Read the model definition and answer for the solid it produces. Units are mm, in the model's axes. Face numbers are marked on the shaded views. A direction names the side the tool comes from. Coordinates: 2 decimals unless noted, no trailing zeros. Write each loop counter-clockwise with the first axis right and the second up, starting at its lowest first coordinate (ties: lowest second). Pieces come first, ordered by that corner, then holes. Notation, with made-up numbers: (-13, -19.75) -> (0, -19.75) arc R26 cw to (0, -5.75) -> close; hole circle Ø11 at (21, 27). An arc over 180 degrees is marked (long way). Answer as a JSON object with one key per item and string values. Group by question number.
(1) Flat-ended cylindrical pins translate along their axes: P1, Ø4, axis at x = 36.5, y = 36, coming from the +Z side; P2, Ø2, axis at x = -17, z = 1, coming from the -Y side; P3, Ø1, axis at y = -8.5, z = 1.5, coming from the -X side. Find the tip coordinate at first contact, or state that the pin passes through.
(2) Find section D-D (z = 6.75). Give the vertices of the cut face in (x, y).
(3) Straight lines are drawn through the part: L1, parallel to Y at x = -37.5, z = 2.5; L2, parallel to Y at x = 37.5, z = 6.75; L3, parallel to X at y = 37.5, z = 3.6. For each, find the intervals that lie inside material, in ascending order.
(4) Find section C-C (z = 1.5). Give the vertices of the cut face in (x, y).
(5) Which of the six approach directions +Z, -Z, +X, -X, +Y, -Y give full straight-line access (tool end or side, diameter ignored) to the marked faces 3 and 4?
(6) For a pull along X with two mould halves and no side action, classify the marked faces 1 and 2 as +X half, -X half, draft (parallel to the pull), parting line (faces both ways), or undercut.
(7) Find section A-A (y = 37.5). Give the vertices of the cut face in (x, z).
(8) Find section B-B (x = -37.5). Give the vertices of the cut face in (y, z).
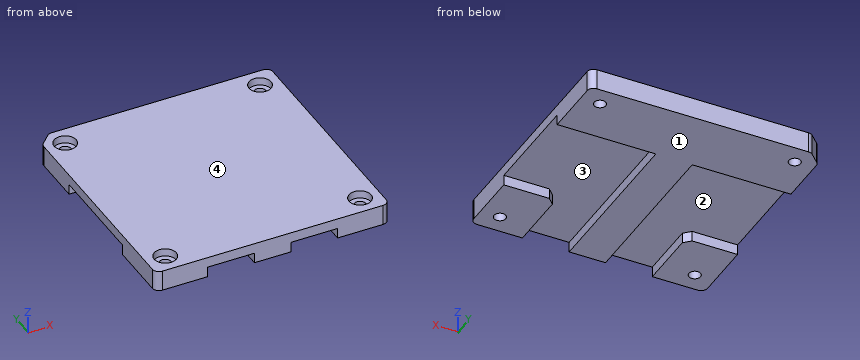
from build123d import *

# Parameters (mm, degrees)
SKETCH_W        = 90
SKETCH_H        = 90
SKETCH_R        = 2.25
PAD_DEPTH       = 8
SKETCH001_R     = 4.25
POCKET_DEPTH    = 3
CHAMFER_SIZE    = 5
POCKET001_DEPTH = 4
FILLET_R        = 2.5
CHAMFER001_SIZE = 2.5


with BuildPart() as part:
    # Sketch → Pad (new body)
    with BuildSketch(Plane.XY):
        Rectangle(SKETCH_W, SKETCH_H)
        with Locations((-37.5, 37.5)):
            Circle(SKETCH_R, mode=Mode.SUBTRACT)
        with Locations((37.5, 37.5)):
            Circle(SKETCH_R, mode=Mode.SUBTRACT)
        with Locations((-37.5, -37.5)):
            Circle(SKETCH_R, mode=Mode.SUBTRACT)
        with Locations((37.5, -37.5)):
            Circle(SKETCH_R, mode=Mode.SUBTRACT)
    extrude(amount=PAD_DEPTH)

    # Sketch001 (on Face10 of Pad) → Pocket (cut)
    with BuildSketch(Plane.XY.offset(8)):
        with Locations((-37.5, 37.5)):
            Circle(SKETCH001_R)
        with Locations((37.5, 37.5)):
            Circle(SKETCH001_R)
        with Locations((-37.5, -37.5)):
            Circle(SKETCH001_R)
        with Locations((37.5, -37.5)):
            Circle(SKETCH001_R)
    extrude(amount=-POCKET_DEPTH, mode=Mode.SUBTRACT)

    # Chamfer
    chamfer_edges = [part.edges().sort_by_distance(p)[0] for p in [
        (-45, 45, 4),
    ]]
    chamfer(chamfer_edges, length=CHAMFER_SIZE)

    # Sketch002 (on Face2 of Chamfer) → Pocket001 (cut)
    with BuildSketch(Plane(origin=(0, 0, 0), x_dir=(1, 0, 0), z_dir=(0, 0, -1))):
        Polygon((-45, 20), (-25, 20), (-25, 45), (-7, 45), (-7, -20), (-45, -20), align=None)
        Polygon((45, 20), (25, 20), (25, 45), (7, 45), (7, -20), (45, -20), align=None)
    extrude(amount=-POCKET001_DEPTH, mode=Mode.SUBTRACT)

    # Fillet
    fillet_edges = [part.edges().sort_by_distance(p)[0] for p in [
        (45, -45, 4),
        (45, 45, 4),
        (-45, -45, 4),
        (-40, 45, 4),
        (-45, 40, 4),
    ]]
    fillet(fillet_edges, radius=FILLET_R)

    # Chamfer001
    chamfer001_edges = [part.edges().sort_by_distance(p)[0] for p in [
        (25, -20, 2),
        (-25, -20, 2),
    ]]
    chamfer(chamfer001_edges, length=CHAMFER001_SIZE)


solid = part.part
Results below:
{
 "1": {"P1": "stops at z = 5", "P2": "stops at y = 20", "P3": "stops at x = -7"},
 "2": {"outline": "(-45, -42.5) arc R2.5 ccw to (-42.5, -45) -> (42.5, -45) arc R2.5 ccw to (45, -42.5) -> (45, 42.5) arc R2.5 ccw to (42.5, 45) -> (-38.96, 45) arc R2.5 ccw to (-40.73, 44.27) -> (-44.27, 40.73) arc R2.5 ccw to (-45, 38.96) -> close; hole circle Ø8.5 at (-37.5, -37.5); hole circle Ø8.5 at (-37.5, 37.5); hole circle Ø8.5 at (37.5, -37.5); hole circle Ø8.5 at (37.5, 37.5)"},
 "3": {"L1": "y = -45 to -39.75, -35.25 to -20, 20 to 35.25, 39.75 to 45", "L2": "y = -45 to -41.75, -33.25 to 33.25, 41.75 to 45", "L3": "x = -45 to -39.75, -35.25 to 35.25, 39.75 to 45"},
 "4": {"outline": "(-45, -42.5) arc R2.5 ccw to (-42.5, -45) -> (-25, -45) -> (-25, -22.5) -> (-27.5, -20) -> (-45, -20) -> close; (-45, 20) -> (-7, 20) -> (-7, -45) -> (7, -45) -> (7, 20) -> (45, 20) -> (45, 42.5) arc R2.5 ccw to (42.5, 45) -> (-38.96, 45) arc R2.5 ccw to (-40.73, 44.27) -> (-44.27, 40.73) arc R2.5 ccw to (-45, 38.96) -> close; (25, -45) -> (42.5, -45) arc R2.5 ccw to (45, -42.5) -> (45, -20) -> (27.5, -20) -> (25, -22.5) -> close; hole circle Ø4.5 at (-37.5, -37.5); hole circle Ø4.5 at (-37.5, 37.5); hole circle Ø4.5 at (37.5, -37.5); hole circle Ø4.5 at (37.5, 37.5)"},
 "5": {"face 3": "-Z", "face 4": "+Z, +X, -X, +Y, -Y"},
 "6": {"face 1": "draft", "face 2": "undercut"},
 "7": {"outline": "(-45, 0) -> (-39.75, 0) -> (-39.75, 5) -> (-41.75, 5) -> (-41.75, 8) -> (-45, 8) -> close; (-35.25, 0) -> (35.25, 0) -> (35.25, 5) -> (33.25, 5) -> (33.25, 8) -> (-33.25, 8) -> (-33.25, 5) -> (-35.25, 5) -> close; (39.75, 0) -> (45, 0) -> (45, 8) -> (41.75, 8) -> (41.75, 5) -> (39.75, 5) -> close"},
 "8": {"outline": "(-45, 0) -> (-39.75, 0) -> (-39.75, 5) -> (-41.75, 5) -> (-41.75, 8) -> (-45, 8) -> close; (-35.25, 0) -> (-20, 0) -> (-20, 4) -> (20, 4) -> (20, 0) -> (35.25, 0) -> (35.25, 5) -> (33.25, 5) -> (33.25, 8) -> (-33.25, 8) -> (-33.25, 5) -> (-35.25, 5) -> close; (39.75, 0) -> (45, 0) -> (45, 8) -> (41.75, 8) -> (41.75, 5) -> (39.75, 5) -> close"}
}
